The listing builds one solid part. Answer for the finished solid, in the listing's coordinates (mm). A direction names the side the tool comes from. Give positions to 0.01 mm unless a question says otherwise; leave off trailing zeros. Loops run counter-clockwise (first coordinate to the right, second up) from the corner with the lowest first, then second, coordinate; pieces in that order, holes last. Notation, with made-up numbers: M -0.5,-40 L 45.5,-40 A18 ccw 45.5,-25 Z; hole C 72.5,55.5 d4. An arc over 180 degrees is marked long. One line per item, written item: value. Start each with the question number.
Q1. Flat-ended cylindrical pins translate along their axes: pin 1 (6 mm diameter, centred on y = -5, z = 18.5, fed in from -X); pin 2 (14 mm diameter, centred on x = -44, y = -17, fed in from +Z); pin 3 (3 mm diameter, centred on x = 7, y = -19, fed in from +Z). Find the tip coordinate at first contact, or state that the pin passes through.
Q2. A cutting plane is placed at C-C, the plane z = 18.25. Determine the outline of the cut face in (x, y), and give its area (3 significant figures).
Q3. The mould has two halves that part along X. Classify faces 5 (the flat face through (8, -13, 0)), 6 (the cylindrical face through (-0.11, -12.52, 5.08)), 7 (the flat face through (-55.281, -13, 6)): +X half, -X half, draft (parallel to the pull), parting line (faces both ways), or undercut.
Q4. For faces 1 (the flat face through (-24, -13, 20.495)), 2 (the flat face through (-23, 0, 9)), 3 (the flat face through (-46, -13, 12.7)), 4 (the flat face through (5, -13, 12.7)), determine the directions among +Z, -Z, +X, -X, +Y, -Y from which every point of the face is accessible in a straight line to the end or side of a thin tool.
Q5. Consider L1, parallel to Z at x = -16, y = -23.5; L2, parallel to X at y = -22.25, z = 3; L3, parallel to X at y = -1.5, z = 14. Determine where each line is inside the solid, lowest interval first.
Q6. A cutting plane is placed at D-D, the plane x = -30. Determine the outline of the cut face in (y, z), and give its area (3 significant figures).
Q7. A cutting plane is placed at B-B, the plane y = -11. Determine the outline of the cut face in (x, z).
Q8. A cutting plane is placed at A-A, the plane x = -12.5. Determine the outline of the cut face in (y, z).
from build123d import *

# Parameters (mm, degrees)
F1_DEPTH = 25.4
F3_DEPTH = 25.4
F4_W     = 9.634385
F4_H     = 7.539335
F5_DEPTH = 25.4
F7_DEPTH = 25.4


with BuildPart() as f1:
    # F0 (on Front) → F1 (new body)
    with BuildSketch(Plane.XZ):
        with BuildLine():
            Line((-37.501371, 12.7), (-55.281371, 12.7))
            Line((-55.281371, 12.7), (-55.281371, 0))
            Line((-55.281371, 0), (-49.858869, 0))
            ThreePointArc((-49.858869, 0), (-44.778869, 5.08), (-39.698869, 0))
            Line((-39.698869, 0), (-5.08, 0))
            ThreePointArc((-5.08, 0), (0, 5.08), (5.08, 0))
            Line((5.08, 0), (10.16, 0))
            Line((10.16, 0), (10.16, 12.7))
            Line((10.16, 12.7), (0, 12.7))
            Line((0, 12.7), (-8.544024, 22.096257))
            Line((-8.544024, 22.096257), (-28.957347, 22.096257))
            Line((-28.957347, 22.096257), (-37.501371, 12.7))
        make_face()
    extrude(amount=F1_DEPTH)

    # F2 (on face) → F3 (cut)
    with BuildSketch(Plane.XZ.offset(25.4)):
        Polygon((-28.253765, 20.494862), (-34.789096, 12.980141), (-20.598149, 12.980141), (-20.598149, 20.494862), align=None)
    extrude(amount=-F3_DEPTH, mode=Mode.SUBTRACT)

    # F4 (on face) → F5 (cut)
    with BuildSketch(Plane.XZ.offset(25.4)):
        with Locations((-14.375965, 16.666421)):
            Rectangle(F4_W, F4_H)
    extrude(amount=-F5_DEPTH, mode=Mode.SUBTRACT)

    # F6 (on face) → F7 (cut)
    with BuildSketch(Plane.XZ.offset(25.4)):
        Polygon((-1.828437, 12.872539), (-8.559588, 20.295901), (-8.559588, 12.872539), align=None)
    extrude(amount=-F7_DEPTH, mode=Mode.SUBTRACT)


solid = f1.part
Answer block:
1. pin 1: x = -34.96
1. pin 2: z = 13.25
1. pin 3: z = 12.7
2. outline: M -32.45,-25.4 L -30.21,-25.4 L -30.21,0 L -32.45,0 Z; M -20.6,-25.4 L -19.19,-25.4 L -19.19,0 L -20.6,0 Z; M -9.56,-25.4 L -8.56,-25.4 L -8.56,0 L -9.56,0 Z; M -6.7,-25.4 L -5.05,-25.4 L -5.05,0 L -6.7,0 Z
2. area: 160 mm^2
3. face 5: draft
3. face 6: undercut
3. face 7: -X half
4. face 1: +Y, -Y
4. face 2: +Z, -Z, +X, -X, +Y
4. face 3: +Z, -X, +Y, -Y
4. face 4: +Z, +X, +Y, -Y
5. L1: 0 to 12.9, 20.44 to 22.1
5. L2: -55.28 to -48.88, -40.68 to -4.1, 4.1 to 10.16
5. L3: -36.32 to -33.9, -20.6 to -19.19, -9.56 to -8.56, -2.85 to -1.18
6. outline: M -25.4,0 L 0,0 L 0,12.98 L -25.4,12.98 Z; M -25.4,18.49 L 0,18.49 L 0,20.95 L -25.4,20.95 Z
6. area: 392 mm^2
7. outline: M -55.28,0 L -49.86,0 A5.08 cw -39.7,0 L -5.08,0 A5.08 cw 5.08,0 L 10.16,0 L 10.16,12.7 L 0,12.7 L -8.54,22.1 L -28.96,22.1 L -37.5,12.7 L -55.28,12.7 Z; hole M -34.79,12.98 L -20.6,12.98 L -20.6,20.49 L -28.25,20.49 Z; hole M -19.19,12.9 L -9.56,12.9 L -9.56,20.44 L -19.19,20.44 Z; hole M -8.56,12.87 L -1.83,12.87 L -8.56,20.3 Z
8. outline: M -25.4,0 L 0,0 L 0,12.9 L -25.4,12.9 Z; M -25.4,20.44 L 0,20.44 L 0,22.1 L -25.4,22.1 Z
